```python
from build123d import *

# Parameters (mm, degrees)
BOSS_EXTRUDE1_DEPTH = 5
SKETCH3_R           = 2.5
CUT_EXTRUDE1_DEPTH  = 5


with BuildPart() as part:
    # Sketch1 → Boss-Extrude1 (new body)
    with BuildSketch(Plane(origin=(0, 0, 0), x_dir=(1, 0, 0), z_dir=(0, 1, 0))):
        with BuildLine():
            Line((-39.418817776, 14.621878605), (10.581182224, 14.621878605))
            ThreePointArc((10.581182224, 14.621878605), (18.081182224, 7.121878605), (10.581182224, -0.378121395))
            Line((10.581182224, -0.378121395), (-39.418817776, -0.378121395))
            ThreePointArc((-39.418817776, -0.378121395), (-46.918817776, 7.121878605), (-39.418817776, 14.621878605))
        make_face()
    extrude(amount=BOSS_EXTRUDE1_DEPTH)

    # Sketch3 → Cut-Extrude1 (cut)
    with BuildSketch(Plane(origin=(0, 5, 0), x_dir=(1, 0, 0), z_dir=(0, 1, 0))):
        with Locations(Location((-39.418817776, 7.121878605, 0), (0, 0, 270))):
            Circle(SKETCH3_R)
        with BuildLine():
            Line((-29.419490327, 9.621878605), (10.581182224, 9.621878605))
            ThreePointArc((10.581182224, 9.621878605), (13.081182224, 7.121878605), (10.581182224, 4.621878605))
            Line((10.581182224, 4.621878605), (-29.419490327, 4.621878605))
            ThreePointArc((-29.419490327, 4.621878605), (-31.919490327, 7.121878605), (-29.419490327, 9.621878605))
        make_face()
    extrude(amount=-CUT_EXTRUDE1_DEPTH, mode=Mode.SUBTRACT)


solid = part.part
```
Model file for the job. Use its own axes, mm. A direction names the side the tool comes from. Give positions to 0.01 mm unless a question says otherwise; leave off trailing zeros. Order: outer loops, then holes, each group sorted by start corner. A loop starts at its lowest first (then second) coordinate and runs counter-clockwise, first axis right, second up.
1) 3-axis set-ups, long thin cutter, end or side, ignore diameter. For faces 1 (the cylindrical face through (13.08, 2.54, -7.18)), 2 (the cylindrical face through (18.08, 2.46, -7.29)): which of +Z, -Z, +X, -X, +Y, -Y reach the whole face in a straight line?
2) Saw through at D-D, the plane x = -31. Write the cut outline in (y, z), then the cut area to 3 significant figures.
3) Saw through at C-C, the plane z = -6.25. Write the cut outline in (x, y).
4) Saw through at A-A, the plane x = 1. Write the cut outline in (y, z), then the cut area to 3 significant figures.
5) Saw through at B-B, the plane y = 0.9. Write the cut outline in (x, z).
6) Pin check, flat tips, straight feed: pin 1 (3 mm diameter, centred on x = -39.42, z = -7.12, fed in from +Y); pin 2 (2 mm diameter, centred on y = 1, z = -4.5, fed in from -X); pin 3 (2 mm diameter, centred on y = 1.5, z = -11.5, fed in from +X). Stop position of each tip, or through.
7) Wall check: probe 1 along Z at (x, y) = (-20, 2.1); probe 2 along X at (y, z) = (0.45, -8.5); probe 3 along X at (y, z) = (4.55, -8.25). Give the ranges that are in metal, low to high.
8) Mould opens along Z. For faces 3 (the flat face through (-14, 5, -4)), 4 (the flat face through (-14, 2, 0.378)), 5 (the flat face through (-9, 3, -4.622)), 6 (the cylindrical face through (-37.31, 2.54, -5.78)) say: +Z half, -Z half, draft (parallel to the pull), parting line (faces both ways), or undercut.
Computed:
1. face 1: +Y, -Y
1. face 2: +X, +Y, -Y
2. outline: (0, -14.62) - (5, -14.62) - (5, -9.06) - (0, -9.06) - close; (0, -5.18) - (5, -5.18) - (5, 0.38) - (0, 0.38) - close
2. area: 55.6 mm2
3. outline: (-46.87, 0) - (-41.76, 0) - (-41.76, 5) - (-46.87, 5) - close; (-37.08, 0) - (-31.76, 0) - (-31.76, 5) - (-37.08, 5) - close; (12.92, 0) - (18.03, 0) - (18.03, 5) - (12.92, 5) - close
4. outline: (0, -14.62) - (5, -14.62) - (5, -9.62) - (0, -9.62) - close; (0, -4.62) - (5, -4.62) - (5, 0.38) - (0, 0.38) - close
4. area: 50.0 mm2
5. outline: (-39.42, -14.62) - (10.58, -14.62) arc R7.5 ccw to (10.58, 0.38) - (-39.42, 0.38) arc R7.5 ccw to start; hole circle Ø5 at (-39.42, -7.12); hole (-29.42, -9.62) - (10.58, -9.62) arc R2.5 ccw to (10.58, -4.62) - (-29.42, -4.62) arc R2.5 ccw to start
6. pin 1: passes through
6. pin 2: stops at x = -46.74
6. pin 3: stops at x = 17.28
7. probe 1: z = -14.62 to -9.62, -4.62 to 0.38
7. probe 2: x = -46.79 to -41.5, -37.33 to -31.51, 12.67 to 17.95
7. probe 3: x = -46.83 to -41.65, -37.19 to -31.65, 12.81 to 18
8. face 3: draft
8. face 4: +Z half
8. face 5: undercut
8. face 6: undercut
